Model file for the job. Use its own axes, mm. A direction names the side the tool comes from. Give positions to 0.01 mm unless a question says otherwise; leave off trailing zeros. Loops run counter-clockwise (first coordinate to the right, second up) from the corner with the lowest first, then second, coordinate; pieces in that order, holes last. Notation, with made-up numbers: M 44.25,28.25 L 103.25,28.25 A25 cw 103.25,56.25 Z; hole C 46.5,48 d2. An arc over 180 degrees is marked long. Answer in a Markdown table with one row per item.
```python
from build123d import *

# Parameters (mm, degrees)
F1_DEPTH = 25.4
F2_DEPTH = 95.758
F3_T     = -2.54
F4_R     = 5.08


with BuildPart() as f1:
    # F0 (on Top) → F1 (new body)
    with BuildSketch(Plane.XY):
        Polygon((-26.5582557768, 28.8428422064), (-50.5463592708, 13.993062079), (-10.2806119248, -17.9910771549), (43.4070453048, -17.9910771549), (12.2796297073, 26.272688061), align=None)
    extrude(amount=F1_DEPTH)

    # F2 (add): a face of the model
    f2_faces = [f1.faces().sort_by_distance(p)[0] for p in [
        (16.56321669, -17.9910771549, 12.7),
    ]]
    extrude(f2_faces, amount=F2_DEPTH)

    # F3
    f3_openings = [f1.faces().sort_by_distance(p)[0] for p in [
        (9.617163, -41.24323, 25.4),
    ]]
    offset(amount=F3_T, openings=f3_openings, kind=Kind.INTERSECTION)

    # F4
    f4_edges = [f1.edges().sort_by_distance(p)[0] for p in [
        (40.867045, -65.001919, 2.54),
        (16.563217, -111.209077, 2.54),
        (-7.740612, -63.98697, 2.54),
        (-26.939148, -1.514961, 2.54),
        (-36.025631, 19.994782, 2.54),
        (-7.506603, 25.036515, 2.54),
        (25.883709, 2.511823, 2.54),
    ]]
    fillet(f4_edges, radius=F4_R)


solid = f1.part
```
(1) Saw through at B-B, the plane y = -39.5. Give the cut face in (x, z).
Established:
| item | result |
|---|---|
| outline | M -10.28,0 L 43.41,0 L 43.41,25.4 L 40.87,25.4 L 40.87,7.62 A5.08 cw 35.79,2.54 L -2.66,2.54 A5.08 cw -7.74,7.62 L -7.74,25.4 L -10.28,25.4 Z |
(2) Saw through at A-A, the plane z = 14.5. Give the cut face in (x, y).
Established:
| item | result |
|---|---|
| outline | M -50.55,13.99 L -10.28,-17.99 L -10.28,-113.75 L 43.41,-113.75 L 43.41,-17.99 L 12.28,26.27 L -26.56,28.84 Z; hole M -46.14,13.73 L -7.74,-16.76 L -7.74,-111.21 L 40.87,-111.21 L 40.87,-18.79 L 10.9,23.82 L -25.91,26.25 Z |
(3) Wall check: L1, parallel to X at y = -87, z = 12; L2, parallel to Z at x = 6, y = -59; L3, parallel to Y at x = -12.5, z = 10.5. Give the ranges that are in metal, low to high.
Established:
| item | result |
|---|---|
| L1 | x = -10.28 to -7.74, 40.87 to 43.41 |
| L2 | z = 0 to 2.54 |
| L3 | y = -16.23 to -12.98, 25.37 to 27.91 |
(4) Flat gauge pins, fed straight in: P1, Ø8, axis at y = -71, z = 19.5, coming from the -X side; P2, Ø1.5, axis at y = -15, z = 10.5, coming from the -X side; P3, Ø5.5, axis at x = 19, z = 17, coming from the +Y side. Where does each tip first touch, or does it go through?
Established:
| item | result |
|---|---|
| P1 | stops at x = -10.28 |
| P2 | stops at x = -14.99 |
| P3 | stops at y = 20.63 |
(5) Mould opens along Y. For faces 3 (the cylindrical face through (-7.35, 23.495, 3.989)), 4 (the flat face through (-10.281, -65, 13)), 5 (the flat face through (-38.384, 21.522, 12.522)) say: pulls with the +Y half, pulls with the -Y half, needs draft (parallel to the pull), parting line crosses it, or undercut.
Established:
| item | result |
|---|---|
| face 3 | undercut |
| face 4 | needs draft |
| face 5 | pulls with the +Y half |
(6) Which spindle directions (+Z, -Z, +X, -X, +Y, -Y) get a long thin tool onto all of the face, cutting with end or side? Do faces 1 (the flat face through (16, -111.209, 16)), 2 (the flat face through (-11, -16, 25.4)). Say none if no direction does.
Established:
| item | result |
|---|---|
| face 1 | +Z |
| face 2 | +Z, +X, -X, +Y, -Y |
